from build123d import *

# Parameters (mm, degrees)
F2_W         = 152.4
F2_H         = 152.4
F3_DEPTH     = 50.8
F5_DEPTH     = 50.8
F6_R         = 152.4
F7_DEPTH     = 25.4
F8_T         = 6.35
F8_T3_DEPTH  = 165.1
F8_T5_DEPTH  = 165.1
F8_T7_DEPTH  = 546.1
F8_T9_DEPTH  = 165.1
F8_T12_ANGLE = 180.000000001
F8_T14_ANGLE = 180.000000001
F9_W         = 101.6
F9_H         = 101.6
F9_R         = 25.4
F10_DEPTH    = 38.1
F11_R        = 19.05


# Not quite as in the source:
# - a pattern or mirror of a feature is missing from the dataset's text; its kind, count and spacing are read off the source's solid
# - a shell that OpenCascade refuses in one call is made with other operations: the cavity is built on its own and cut out


with BuildPart() as f1:
    # F0 (on Front) → F1 (revolve)
    with BuildSketch(Plane.XZ):
        Polygon((-101.6, 0), (0, 0), (0, 1295.4), (-482.6, 1295.4), (-533.4, 1244.6), (-533.4, 431.8), align=None)
    revolve(axis=Axis((0, 0, 647.7), (0, 0, -1)))

    # F2 (on face) → F3 (join)
    with BuildSketch(Plane.XY.offset(1295.4)):
        with Locations((381, 0)):
            Rectangle(F2_W, F2_H)
    f3 = extrude(amount=F3_DEPTH)

    # F3_copies: F3 across plane
    add(f3.mirror(Plane(origin=(0, 0, 0), x_dir=(0, 0, -1), z_dir=(-1, 0, 0))))

    # F4 (on face) → F5 (join)
    with BuildSketch(Plane.XY.offset(1295.4)):
        with BuildLine():
            ThreePointArc((0, 463.55), (-139.1939698766, 405.8939698766), (-196.85, 266.7))
            Line((-196.85, 266.7), (-196.85, -266.7))
            ThreePointArc((-196.85, -266.7), (-139.1939698766, -405.8939698766), (0, -463.55))
            ThreePointArc((0, -463.55), (139.1939698766, -405.8939698766), (196.85, -266.7))
            Line((196.85, -266.7), (196.85, 266.7))
            ThreePointArc((196.85, 266.7), (139.1939698766, 405.8939698766), (0, 463.55))
        make_face()
    extrude(amount=F5_DEPTH)

    # F6 (on face) → F7 (cut)
    with BuildSketch(Plane.XY.offset(1346.2)):
        with Locations((0, -266.7)):
            Circle(F6_R)
    extrude(amount=-F7_DEPTH, mode=Mode.SUBTRACT)

    # F8: shell of thickness 6.35, made by hand


with BuildPart() as f8_core1:
    # F8_t2: copy of F1
    add(f1.part)

    # the walls: a layer under each face that stays
    f8_faces = [f8_core1.faces().sort_by_distance(p)[0] for p in [
        (0, 0, 0),
        (317.5, 0, 215.9),
        (533.4, 0, 838.2),
        (508, 0, 1270),
        (-321.7333333333, -321.7333333333, 1295.4),
        (-457.2, 0, 1320.8),
        (-381, -76.2, 1320.8),
        (-381, 76.2, 1320.8),
        (-304.8, 0, 1320.8),
        (0, 463.55, 1320.8),
        (-196.85, 0, 1320.8),
        (0, -463.55, 1320.8),
        (196.85, 0, 1320.8),
        (381, 76.2, 1320.8),
        (457.2, 0, 1320.8),
        (304.8, 0, 1320.8),
        (381, -76.2, 1320.8),
        (-381, 0, 1346.2),
        (0, 0, 1346.2),
        (381, 0, 1346.2),
        (-152.4, -266.7, 1333.5),
    ]]
    thicken(f8_faces, amount=-F8_T, mode=Mode.SUBTRACT)

    # F8_s4 → F8_t3 (cut)
    with BuildSketch(Plane.XZ.offset(-82.55)):
        Polygon((-457.2635, 1295.4635), (-457.2, 1289.05), (-450.85, 1289.05), (-450.85, 1295.4), align=None)
        Polygon((-304.7365, 1295.4635), (-304.8, 1289.05), (-311.15, 1289.05), (-311.15, 1295.4), align=None)
        Polygon((457.2635, 1295.4635), (457.2, 1289.05), (450.85, 1289.05), (450.85, 1295.4), align=None)
        Polygon((304.7365, 1295.4635), (304.8, 1289.05), (311.15, 1289.05), (311.15, 1295.4), align=None)
    extrude(amount=F8_T3_DEPTH, mode=Mode.SUBTRACT)

    # F8_s6 → F8_t5 (cut)
    with BuildSketch(Plane.YZ.offset(-463.55)):
        Polygon((-76.2635, 1295.4635), (-76.2, 1289.05), (-69.85, 1289.05), (-69.85, 1295.4), align=None)
        Polygon((76.2635, 1295.4635), (76.2, 1289.05), (69.85, 1289.05), (69.85, 1295.4), align=None)
    extrude(amount=F8_T5_DEPTH, mode=Mode.SUBTRACT)

    # F8_s8 → F8_t7 (cut)
    with BuildSketch(Plane.XZ.offset(-273.05)):
        Polygon((-196.9135, 1295.4635), (-196.85, 1289.05), (-190.5, 1289.05), (-190.5, 1295.4), align=None)
        Polygon((196.9135, 1295.4635), (196.85, 1289.05), (190.5, 1289.05), (190.5, 1295.4), align=None)
    extrude(amount=F8_T7_DEPTH, mode=Mode.SUBTRACT)

    # F8_s10 → F8_t9 (cut)
    with BuildSketch(Plane.YZ.offset(298.45)):
        Polygon((76.2635, 1295.4635), (76.2, 1289.05), (69.85, 1289.05), (69.85, 1295.4), align=None)
        Polygon((-76.2635, 1295.4635), (-76.2, 1289.05), (-69.85, 1289.05), (-69.85, 1295.4), align=None)
    extrude(amount=F8_T9_DEPTH, mode=Mode.SUBTRACT)

    # F8_s11 → F8_t12 (revolve, cut)
    with BuildSketch(Plane.XZ.offset(-266.7)):
        Polygon((196.9135, 1295.4635), (196.85, 1289.05), (190.5, 1289.05), (190.5, 1295.4), align=None)
    revolve(axis=Axis((0, 266.7, 1295.4), (0, 0, 1)), revolution_arc=F8_T12_ANGLE, mode=Mode.SUBTRACT)

    # F8_s13 → F8_t14 (revolve, cut)
    with BuildSketch(Plane.XZ.offset(266.7)):
        Polygon((-196.9135, 1295.4635), (-196.85, 1289.05), (-190.5, 1289.05), (-190.5, 1295.4), align=None)
    revolve(axis=Axis((0, -266.7, 1295.4), (0, 0, 1)), revolution_arc=F8_T14_ANGLE, mode=Mode.SUBTRACT)


with BuildPart() as f1_1:
    add(f1.part)

    # what is left inside the walls is the cavity
    f8_cavity = [f8_core1.part.solids().sort_by_distance(p)[0] for p in [
        (526.9865, 0, 972.789915),
    ]]
    add(f8_cavity, mode=Mode.SUBTRACT)

    # F9 (on face) → F10 (join)
    with BuildSketch(Plane.XY.offset(6.35)):
        Rectangle(F9_W, F9_H)
        Circle(F9_R, mode=Mode.SUBTRACT)
    extrude(amount=F10_DEPTH)

    # F11
    f11_edges = [f1_1.edges().sort_by_distance(p)[0] for p in [
        (-50.8, -50.8, 25.4),
        (50.8, -50.8, 25.4),
        (50.8, 50.8, 25.4),
        (-50.8, 50.8, 25.4),
    ]]
    fillet(f11_edges, radius=F11_R)


solid = f1_1.part
Geometry: final body of the model. Coordinates: model frame, mm. A direction names the side the tool comes from. Give positions to 0.01 mm unless a question says otherwise; leave off trailing zeros. Write each loop counter-clockwise with the first axis right and the second up, starting at its lowest first coordinate (ties: lowest second). Pieces come first, ordered by that corner, then holes. Notation, with made-up numbers: (-23, 74) -> (-8, 74) arc R26 cw to (-8, 110) -> close; hole circle Ø8 at (27, 29.5). An arc over 180 degrees is marked (long way). Answer as a JSON object with one key per item and string values.
1. Access query for faces 4 (the cylindrical face through (4.329, 463.502, 1320.444)), 5 (the flat face through (-380, 76.2, 1320)), 6 (the flat face through (-311.15, 1, 1314)), 7 (the flat face through (208, 7, 1295.4)). Directions: +Z, -Z, +X, -X, +Y, -Y. A direction counts if a zero-diameter tool reaches every point of the face in a straight line with its end or side. Return the directions, or none.
Ans:
{"face 4": "+Z, +Y", "face 5": "+Z, -X, +Y", "face 6": "none", "face 7": "+Z"}
2. Mould query, pull axis Y, two halves, no side actions, for faces 1 (the flat face through (-380, 1, 1346.2)), 2 (the cylindrical face through (-4.189, -457.154, 1314.806)), 3 (the cylindrical face through (-4.329, -463.502, 1320.444)). Classes: pulls with the +Y half, pulls with the -Y half, needs draft (parallel to the pull), parting line crosses it, or undercut.
Ans:
{"face 1": "needs draft", "face 2": "undercut", "face 3": "pulls with the -Y half"}
3. Contact query for flat-ended pins moving along their axis: pin 1 (15 mm diameter, centred on y = -112, z = 1322.5, fed in from +X); pin 2 (6 mm diameter, centred on y = -126.5, z = 511, fed in from +X); pin 3 (4 mm diameter, centred on x = 167, z = 879.5, fed in from +Y). Output: stop coordinate, or through.
Ans:
{"pin 1": "stops at x = 196.85", "pin 2": "stops at x = 518.91", "pin 3": "stops at y = 507.24"}
4. Ray query, probe 1 along Y at (x, z) = (0, 1335.25); probe 2 along Y at (x, z) = (0, 772.5); probe 3 along Y at (x, z) = (55.5, 1056). Return the intervals inside material, ascending. Write a range as from..to.
Ans:
{"probe 1": "y = -463.55..-457.2, -425.45..-419.1, -114.3..-107.95, 457.2..463.55", "probe 2": "y = -533.4..-527.05, 527.05..533.4", "probe 3": "y = -530.5..-524.12, 524.12..530.5"}
5. Cut plane A-A on z = 1203.5. Output: boundary loops of the cut face in (x, y).
Ans:
{"outline": "circle Ø1066.8 at (0, 0); hole circle Ø1054.1 at (0, 0)"}
